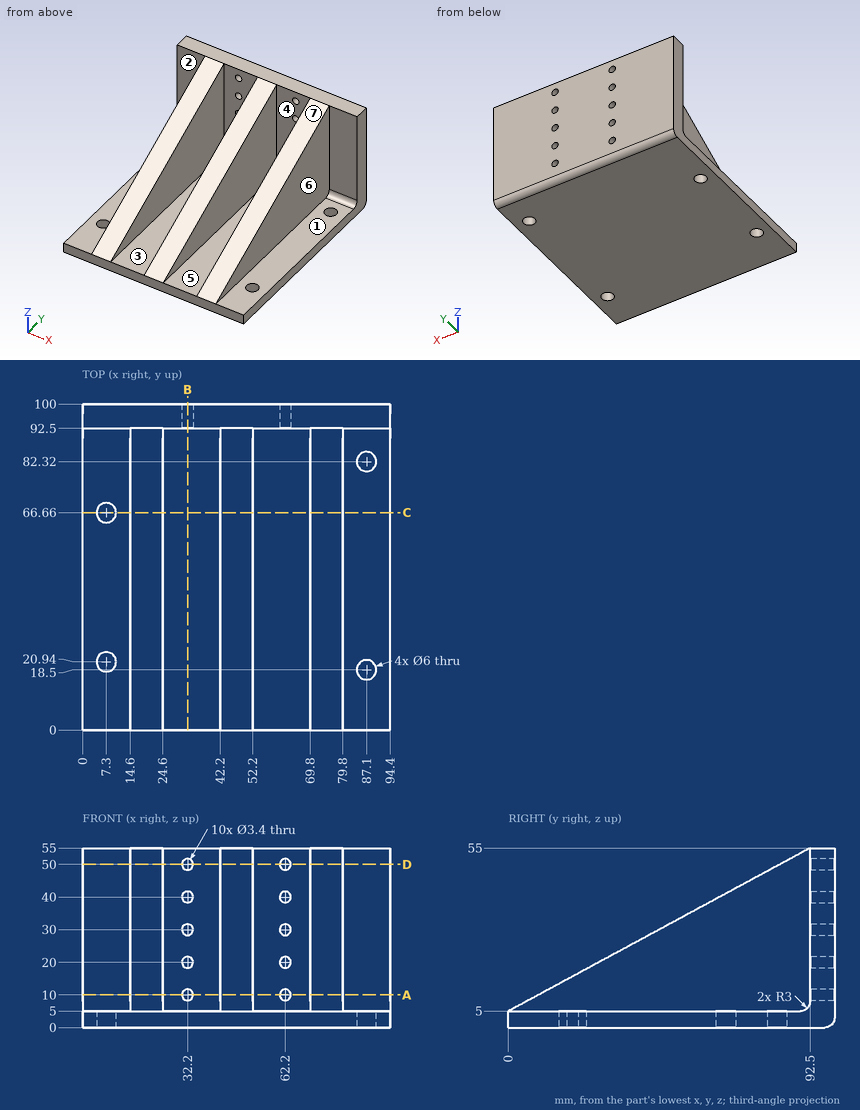
Could you check a few things on this drawing? It's one solid part, dimensions in mm from its lowest x, y, z. A direction names the side the tool comes from. Round coordinates to 2 decimals unless told otherwise and drop trailing zeros. Loops run counter-clockwise (first coordinate to the right, second up) from the corner with the lowest first, then second, coordinate; pieces in that order, holes last. Notation, with made-up numbers: (-35.5, -30.75) -> (-23.5, -30.75) arc R19 ccw to (-23.5, -3.75) -> close; hole circle Ø8 at (43, 20). An arc over 180 degrees is marked (long way). Answer as CSV lines item,"result".
1. Thinking about a two-plate mould opening in X: for the marked faces 4, 5, 6 and 7, which applies, released by +X, released by -X, zero draft, split by the parting line, or undercut?
Final values:
face 4,"undercut"
face 5,"undercut"
face 6,"released by +X"
face 7,"zero draft"
2. If we section it at B-B on x = 32.2: Please give me the cut outline in (y, z).
Final values:
outline,"(0, 0) -> (97, 0) arc R3 ccw to (100, 3) -> (100, 8.3) -> (92.5, 8.3) -> (92.5, 8) arc R3 cw to (89.5, 5) -> (0, 5) -> close; (92.5, 11.7) -> (100, 11.7) -> (100, 18.3) -> (92.5, 18.3) -> close; (92.5, 21.7) -> (100, 21.7) -> (100, 28.3) -> (92.5, 28.3) -> close; (92.5, 31.7) -> (100, 31.7) -> (100, 38.3) -> (92.5, 38.3) -> close; (92.5, 41.7) -> (100, 41.7) -> (100, 48.3) -> (92.5, 48.3) -> close; (92.5, 51.7) -> (100, 51.7) -> (100, 55) -> (92.5, 55) -> close"
3. If we section it at A-A on z = 10: Please give me the cut outline in (x, y), plus the area to 3 significant figures.
Final values:
outline,"(0, 92.5) -> (14.6, 92.5) -> (14.6, 9.25) -> (24.6, 9.25) -> (24.6, 92.5) -> (30.5, 92.5) -> (30.5, 100) -> (0, 100) -> close; (33.9, 92.5) -> (42.2, 92.5) -> (42.2, 9.25) -> (52.2, 9.25) -> (52.2, 92.5) -> (60.5, 92.5) -> (60.5, 100) -> (33.9, 100) -> close; (63.9, 92.5) -> (69.8, 92.5) -> (69.8, 9.25) -> (79.8, 9.25) -> (79.8, 92.5) -> (94.4, 92.5) -> (94.4, 100) -> (63.9, 100) -> close"
area,"3,150 mm^2"
4. If I drill on L1, parallel to X at y = 65, z = 32.5; L2, parallel to Y at x = 7.3, z = 3.95; L3, parallel to X at y = 95.5, z = 50, over which ranges is the centre line in solid material (lowest first)?
Final values:
L1,"x = 14.6 to 24.6, 42.2 to 52.2, 69.8 to 79.8"
L2,"y = 0 to 17.94, 23.94 to 63.66, 69.66 to 100"
L3,"x = 0 to 30.5, 33.9 to 60.5, 63.9 to 94.4"
5. If we section it at C-C on y = 66.66: Please give me the cut outline in (x, z), plus the area to 3 significant figures.
Final values:
outline,"(0, 0) -> (4.3, 0) -> (4.3, 5) -> (0, 5) -> close; (10.3, 0) -> (94.4, 0) -> (94.4, 5) -> (79.8, 5) -> (79.8, 41.03) -> (69.8, 41.03) -> (69.8, 5) -> (52.2, 5) -> (52.2, 41.03) -> (42.2, 41.03) -> (42.2, 5) -> (24.6, 5) -> (24.6, 41.03) -> (14.6, 41.03) -> (14.6, 5) -> (10.3, 5) -> close"
area,"1,520 mm^2"
6. If we section it at D-D on z = 50: Please give me the cut outline in (x, y), plus the area to 4 significant figures.
Final values:
outline,"(0, 92.5) -> (14.6, 92.5) -> (14.6, 83.25) -> (24.6, 83.25) -> (24.6, 92.5) -> (30.5, 92.5) -> (30.5, 100) -> (0, 100) -> close; (33.9, 92.5) -> (42.2, 92.5) -> (42.2, 83.25) -> (52.2, 83.25) -> (52.2, 92.5) -> (60.5, 92.5) -> (60.5, 100) -> (33.9, 100) -> close; (63.9, 92.5) -> (69.8, 92.5) -> (69.8, 83.25) -> (79.8, 83.25) -> (79.8, 92.5) -> (94.4, 92.5) -> (94.4, 100) -> (63.9, 100) -> close"
area,"934.5 mm^2"
7. Which directions (+Z, -Z, +X, -X, +Y, -Y) give clear straight access to the entire face, cutting with the end or side of a thin tool? Please do the marked faces 1, 2 and 3.
Final values:
face 1,"+Z, +X, -Y"
face 2,"+Z, -X, -Y"
face 3,"+Z, -Y"
8. For pin 1 (9 mm diameter, centred on x = 32, z = 42, fed in from -Y); pin 2 (2 mm diameter, centred on y = 29.5, z = 12, fed in from +X); pin 3 (5 mm diameter, centred on x = 41.5, z = 47, fed in from -Y), each with a flat end and sliding along its axis, tell me the tip position at first contact or that it passes through.
Final values:
pin 1,"stops at y = 92.5"
pin 2,"stops at x = 79.8"
pin 3,"stops at y = 73.26"
